from build123d import *

# Parameters (mm, degrees)
F0_R           = 4
F0_W           = 15
F0_H           = 15
F1_DEPTH       = 10
F3_DEPTH       = 25
F5_DEPTH       = 25
F6_SIZE2       = 2.5
F6_SIZE        = 15
F6_2_SIZE2     = 2.5
F6_2_SIZE      = 15
F9_D           = 3
F9_DEPTH       = 10
F9_TIP         = 0.9012909285
F9_ON_F7_D     = 3
F9_ON_F7_DEPTH = 10
F9_ON_F7_TIP   = 0.9012909285


with BuildPart() as f1:
    # F0 (on Top) → F1 (new body)
    with BuildSketch(Plane.XY):
        Polygon((59.23548, -2.5), (39.23548, -2.5), (31.73548, -2.5), (24.23548, -2.5), (4.23548, -2.5), (4.23548, -18.87192), (15.86774, -18.87192), (59.23548, -18.87192), align=None)
        with Locations((31.73548, -10.68596)):
            Circle(F0_R, mode=Mode.SUBTRACT)
        Polygon((39.23548, -2.5), (39.23548, 0), (24.23548, 0), (24.23548, -2.5), (31.73548, -2.5), align=None)
        with Locations((31.73548, 7.5)):
            Rectangle(F0_W, F0_H)
        with Locations((31.73548, 7.5)):
            Circle(F0_R, mode=Mode.SUBTRACT)
    extrude(amount=F1_DEPTH)

    # F2 (on face) → F3 (cut)
    with BuildSketch(Plane.XY.offset(10)):
        Polygon((44.23548, -2.5), (59.23548, -8.18596), (59.23548, -2.5), align=None)
        Polygon((59.23548, -18.87192), (59.23548, -13.18596), (44.23548, -18.87192), align=None)
    extrude(amount=-F3_DEPTH, mode=Mode.SUBTRACT)

    # F4 (on face) → F5 (cut)
    with BuildSketch(Plane.XY.offset(10)):
        Polygon((19.23548, -2.5), (4.23548, -2.5), (4.23548, -8.18596), align=None)
        Polygon((4.23548, -18.87192), (19.23548, -18.87192), (4.23548, -13.18596), align=None)
    extrude(amount=-F5_DEPTH, mode=Mode.SUBTRACT)

    # F6
    f6_edges = [f1.edges().sort_by_distance(p)[0] for p in [
        (4.23548, -10.68596, 10),
        (59.23548, -10.68596, 10),
    ]]
    f6_side = f1.faces().sort_by_distance((51.506527, -5.946976, 10))[0]
    chamfer(f6_edges, length=F6_SIZE, length2=F6_SIZE2, reference=f6_side)

    # F6#2
    f6_2_edges = [f1.edges().sort_by_distance(p)[0] for p in [
        (4.23548, -10.68596, 0),
        (59.23548, -10.68596, 0),
    ]]
    f6_2_side = f1.faces().sort_by_distance((51.506527, -5.946976, 0))[0]
    chamfer(f6_2_edges, length=F6_2_SIZE, length2=F6_2_SIZE2, reference=f6_2_side)

    # F9
    with Locations(Plane.YZ.offset(59.23548)):
        with Locations((-10.68596, 5)):
            Hole(F9_D / 2, depth=F9_DEPTH)
            with Locations((0, 0, -(F9_DEPTH + F9_TIP / 2))):  # 118° drill point
                Cone(0, F9_D / 2, F9_TIP, mode=Mode.SUBTRACT)

    # F9 on F7
    with Locations(Plane(origin=(4.23548, 0, 0), x_dir=(0, -1, 0), z_dir=(-1, 0, 0))):
        with Locations((10.68596, 5)):
            Hole(F9_ON_F7_D / 2, depth=F9_ON_F7_DEPTH)
            with Locations((0, 0, -(F9_ON_F7_DEPTH + F9_ON_F7_TIP / 2))):  # 118° drill point
                Cone(0, F9_ON_F7_D / 2, F9_ON_F7_TIP, mode=Mode.SUBTRACT)


solid = f1.part
Input: part model. Units: mm. Frame: model coordinates. A direction names the side the tool comes from. Coordinates: 2 decimals unless noted, no trailing zeros. Order: outer loops, then holes, each group sorted by start corner. A loop starts at its lowest first (then second) coordinate and runs counter-clockwise, first axis right, second up. Notation, with made-up numbers: M -21.5,11.5 L -7.5,11.5 A31 ccw -7.5,41.5 Z; hole C 11,-1 d9. An arc over 180 degrees is marked long. Answer as CSV lines item,"result".
1. Section A-A (y = 7.5). Return the cut outline in (x, z), then the cut area to 3 significant figures.
Reported:
outline,"M 24.24,0 L 27.74,0 L 27.74,10 L 24.24,10 Z; M 35.74,0 L 39.24,0 L 39.24,10 L 35.74,10 Z"
area,"70.0 mm2"
2. Material intervals for line 1 (X direction, y = -1, z = 5.5); line 2 (Y direction, x = 10.75, z = 5); line 3 (Y direction, x = 10.25, z = 5), sorted ascending. Write a range as from..to.
Reported:
line 1,"24.24..39.24"
line 2,"-15.66..-12.19, -9.19..-5.72"
line 3,"-15.47..-12.19, -9.19..-5.91"
3. Section D-D (x = 13). Return the cut outline in (y, z).
Reported:
outline,"M -16.51,1.04 L -4.86,1.04 L -4.86,8.96 L -16.51,8.96 Z; hole C -10.69,5 d3"
4. Access query for faces 1 (the flat face through (39.235, 6, 5)), 2 (the cylindrical face through (9.305, -12.185, 5.066)), 3 (the cylindrical face through (35.43, -12.22, 4.93)), 4 (the flat face through (22, -2.5, 5)), 5 (the flat face through (13.51, -16.7, 5.07)). Directions: +Z, -Z, +X, -X, +Y, -Y. A direction counts if a zero-diameter tool reaches every point of the face in a straight line with its end or side. Return the directions, or none.
Reported:
face 1,"+Z, -Z, +X, +Y"
face 2,"-X"
face 3,"+Z, -Z"
face 4,"+Z, -Z, -X, +Y"
face 5,"+Z, -Z, -X, -Y"
5. First-contact query: P1, Ø5, axis at x = 31.74, y = -10.69, coming from the -Z side; P2, Ø5, axis at y = 1.5, z = 3, coming from the -X side; P3, Ø1, axis at x = 42, z = 5.5, coming from the +Y side. Flat tips, straight axial feed; report the tip coordinate or a pass-through.
Reported:
P1,"through"
P2,"x = 24.24"
P3,"y = -2.5"
6. Section C-C (x = 29.5). Return the cut outline in (y, z).
Reported:
outline,"M -18.87,0 L -14,0 L -14,10 L -18.87,10 Z; M -7.37,0 L 4.18,0 L 4.18,10 L -7.37,10 Z; M 10.82,0 L 15,0 L 15,10 L 10.82,10 Z"
7. Section B-B (z = 9). Return the cut outline in (x, y), then the cut area to 3 significant figures.
Reported:
outline,"M 13.24,-16.6 L 19.24,-18.87 L 44.24,-18.87 L 50.24,-16.6 L 50.24,-4.77 L 44.24,-2.5 L 39.24,-2.5 L 39.24,15 L 24.24,15 L 24.24,-2.5 L 19.24,-2.5 L 13.24,-4.77 Z; hole C 31.74,-10.69 d8; hole C 31.74,7.5 d8"
area,"740 mm2"
8. Pull-direction query (Y, two-part tool) for faces 6 (the cylindrical face through (54.165, -12.072, 4.425)), 7 (the flat face through (50.174, -16.621, 5.07)), 8 (the flat face through (13.3, -4.75, 5.07)); classes: released by +Y, released by -Y, zero draft, split by the parting line, or undercut.
Reported:
face 6,"undercut"
face 7,"released by -Y"
face 8,"released by +Y"
